Here's the drawing with two shaded views (mm, measured from the low corner). I have some questions. A direction names the side the tool comes from. Round coordinates to 2 decimals unless told otherwise and drop trailing zeros. Write each loop counter-clockwise with the first axis right and the second up, starting at its lowest first coordinate (ties: lowest second). Pieces come first, ordered by that corner, then holes.
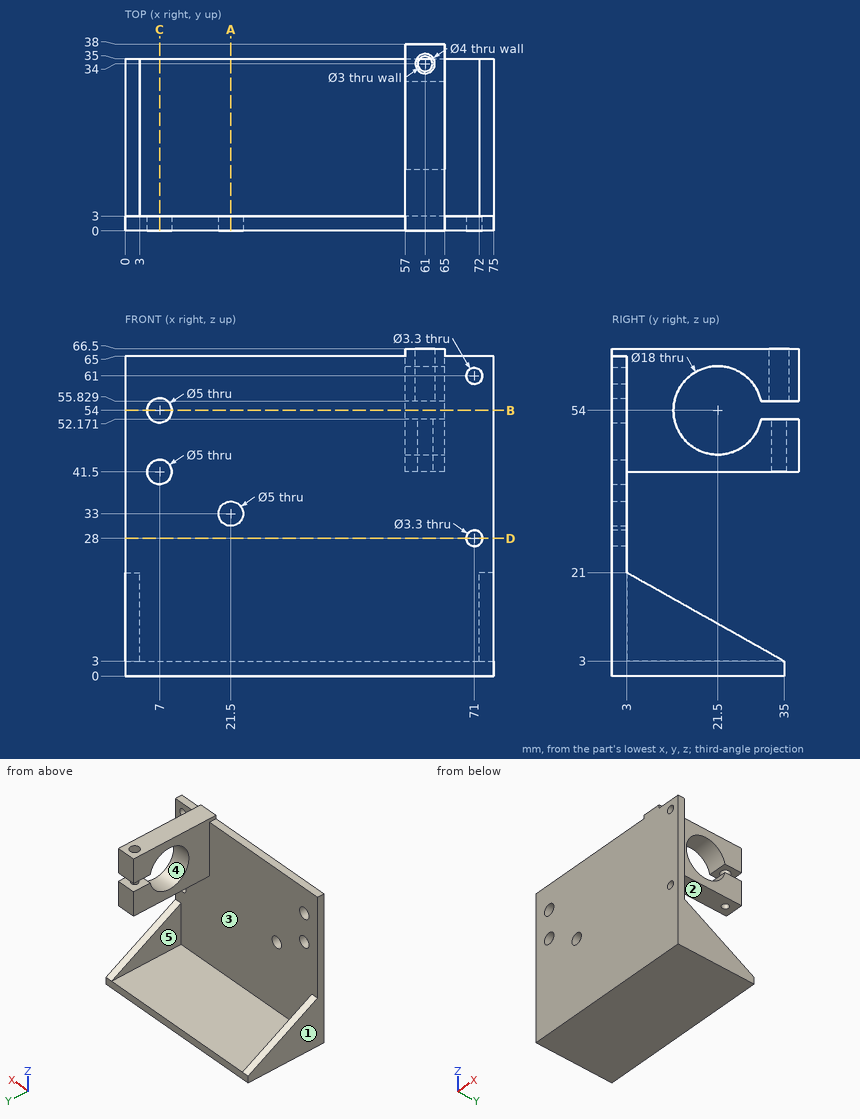
Q1. I'm going to push flat-ended pins straight in: pin 1 Ø3.5 at (x, y) = (69, 2) entering from +Z; pin 2 Ø5.5 at (x, z) = (71, 61) entering from +Y; pin 3 Ø12 at (x, y) = (14, 30) entering from -Z; pin 4 Ø1 at (y, z) = (11.5, 49) entering from +X. Where does each tip first touch, or does it pass through?
Q2. We'd pull the mould along Y, two halves only. Please class the marked faces 3, 4 and 5: pulls with the +Y half, pulls with the -Y half, needs draft (parallel to the pull), parting line crosses it, or undercut.
Q3. On a 3-axis mill with a long thin cutter (end or side, diameter ignored), from which of +Z, -Z, +X, -X, +Y, -Y can I reach the whole of each face in a straight line? I mean the marked faces 1 and 2. Say none if no direction works.
Q4. Imagine slicing it at B-B, the plane z = 54. Write out the boundary of the cut face in (x, y), then the cut area to 3 significant figures.
Q5. If I drill on L1, parallel to X at y = 2, z = 54; L2, parallel to Z at x = 60, y = 5.5; L3, parallel to Z at x = 7, y = 1, over which ranges is the centre line in solid material (lowest first)?
Q6. Imagine slicing it at A-A, the plane x = 21.5. Write out the boundary of the cut face in (y, z), then the cut area to 3 significant figures.
Q7. Imagine slicing it at C-C, the plane x = 7. Write out the boundary of the cut face in (y, z), then the cut area to 3 significant figures.
Q8. Imagine slicing it at D-D, the plane z = 28. Write out the boundary of the cut face in (x, y).
Results found:
1. pin 1: stops at z = 65
1. pin 2: stops at y = 3
1. pin 3: stops at z = 0
1. pin 4: stops at x = 65
2. face 3: pulls with the +Y half
2. face 4: undercut
2. face 5: needs draft
3. face 1: +Z, -Z, -X, +Y, -Y
3. face 2: +X, -X, +Y
4. outline: (0, 0) - (4.5, 0) - (4.5, 3) - (0, 3) - close; (9.5, 0) - (75, 0) - (75, 3) - (65, 3) - (65, 12.5) - (57, 12.5) - (57, 3) - (9.5, 3) - close
4. area: 286 mm2
5. L1: x = 0 to 4.5, 9.5 to 75
5. L2: z = 0 to 3, 41.5 to 66.5
5. L3: z = 0 to 39, 44 to 51.5, 56.5 to 65
6. outline: (0, 0) - (35, 0) - (35, 3) - (3, 3) - (3, 30.5) - (0, 30.5) - close; (0, 35.5) - (3, 35.5) - (3, 65) - (0, 65) - close
6. area: 276 mm2
7. outline: (0, 0) - (35, 0) - (35, 3) - (3, 3) - (3, 39) - (0, 39) - close; (0, 44) - (3, 44) - (3, 51.5) - (0, 51.5) - close; (0, 56.5) - (3, 56.5) - (3, 65) - (0, 65) - close
7. area: 261 mm2
8. outline: (0, 0) - (69.35, 0) - (69.35, 3) - (0, 3) - close; (72.65, 0) - (75, 0) - (75, 3) - (72.65, 3) - close
